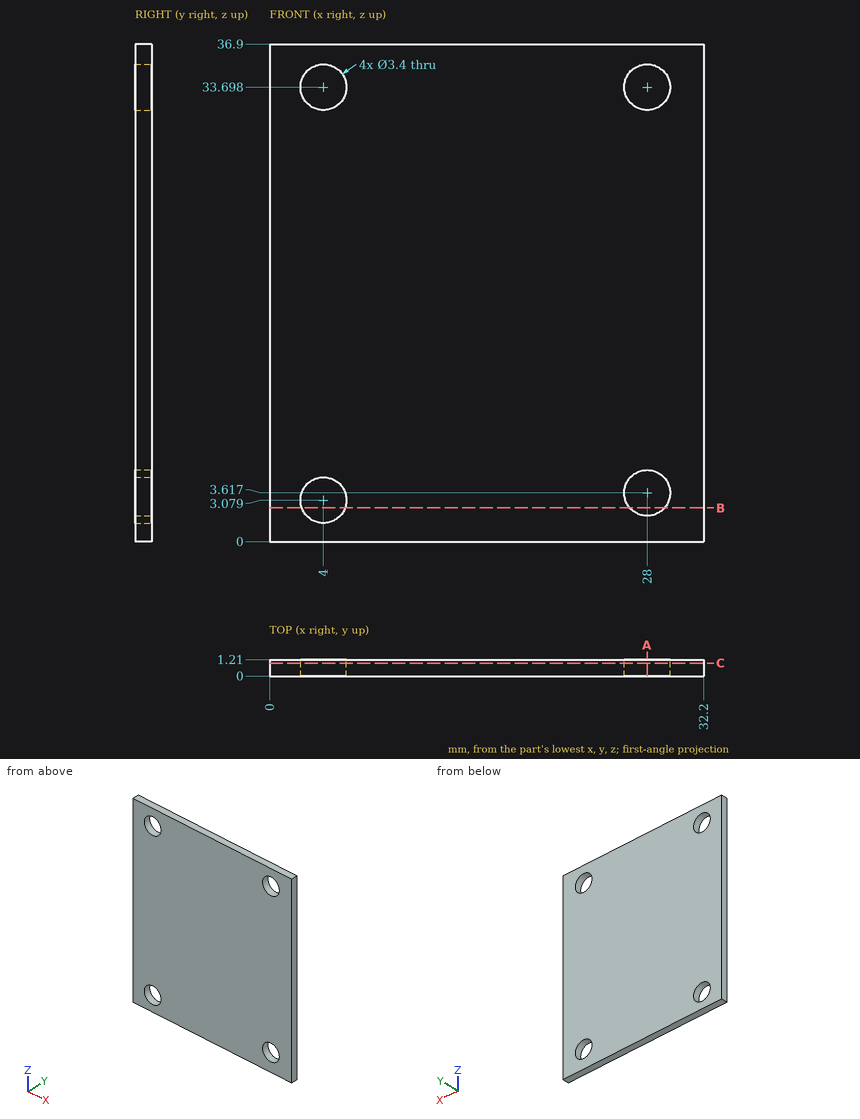
Here's the drawing with two shaded views (mm, measured from the low corner). I have some questions. Coordinates: 2 decimals unless noted, no trailing zeros. Write each loop counter-clockwise with the first axis right and the second up, starting at its lowest first coordinate (ties: lowest second). Pieces come first, ordered by that corner, then holes. Notation, with made-up numbers: (-8.5, 28) -> (29.5, 28) arc R17 cw to (29.5, 48) -> close; hole circle Ø11 at (36, -36). An arc over 180 degrees is marked (long way). Write item = value, one per line. Start each with the question number.
(1) I need wall thicknesses on line 1 (Z direction, x = 4, y = 0.4); line 2 (Z direction, x = 28, y = 0.7); line 3 (X direction, y = 0.4, z = 4) (1 decimal). Which ranges of each line are inside material? Lowest first, please. Write a range as [from, to].
(2) I want a section at C-C (y = 0.95). Please give me the cut outline in (x, z).
(3) I want a section at A-A (x = 28). Please give me the cut outline in (y, z).
(4) I want a section at B-B (z = 2.5). Please give me the cut outline in (x, y).
Result set:
q1.line_1 = [0, 1.38], [4.78, 32], [35.4, 36.9]
q1.line_2 = [0, 1.92], [5.32, 32], [35.4, 36.9]
q1.line_3 = [0, 2.6], [5.4, 26.3], [29.7, 32.2]
q2.outline = (0, 0) -> (32.2, 0) -> (32.2, 36.9) -> (0, 36.9) -> close; hole circle Ø3.4 at (4, 3.08); hole circle Ø3.4 at (4, 33.7); hole circle Ø3.4 at (28, 3.62); hole circle Ø3.4 at (28, 33.7)
q3.outline = (0, 0) -> (1.21, 0) -> (1.21, 1.92) -> (0, 1.92) -> close; (0, 5.32) -> (1.21, 5.32) -> (1.21, 32) -> (0, 32) -> close; (0, 35.4) -> (1.21, 35.4) -> (1.21, 36.9) -> (0, 36.9) -> close
q4.outline = (0, 0) -> (2.4, 0) -> (2.4, 1.21) -> (0, 1.21) -> close; (5.6, 0) -> (26.72, 0) -> (26.72, 1.21) -> (5.6, 1.21) -> close; (29.28, 0) -> (32.2, 0) -> (32.2, 1.21) -> (29.28, 1.21) -> close
